Here's how the part is built. I have some questions about the finished solid (model axes, mm). Round coordinates to 2 decimals unless told otherwise and drop trailing zeros. Loops run counter-clockwise (first coordinate to the right, second up) from the corner with the lowest first, then second, coordinate; pieces in that order, holes last. Notation, with made-up numbers: M -31.75,-37.5 L -16.75,-37.5 A29 cw -16.75,-13.5 Z; hole C -12,41 d8. An arc over 180 degrees is marked long. Use a Markdown table: item, result.
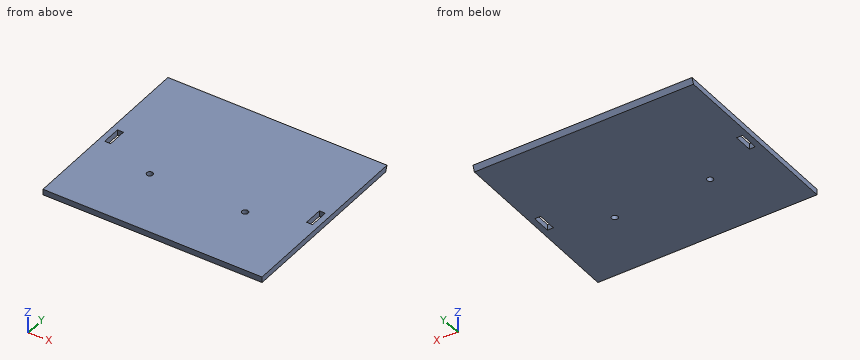
from build123d import *

# Parameters (mm, degrees)
F0_W     = 115
F0_H     = 98
F1_DEPTH = 3
F2_W     = 3.1
F2_H     = 10
F3_DEPTH = 3
F4_SIZE2 = 1.091901
F4_SIZE  = 2.99999
F8_D     = 3.2
F8_DEPTH = 5
F8_TIP   = 0.9613769904


# Not quite as in the source:
# - a fillet or chamfer is up to 0.001 mm smaller than in the source, because OpenCascade refuses the exact size
# - a pattern or mirror of a feature is missing from the dataset's text; its kind, count and spacing are read off the source's solid


with BuildPart() as f1:
    # F0 (on Top) → F1 (new body)
    with BuildSketch(Plane.XY):
        Rectangle(F0_W, F0_H)
    extrude(amount=-F1_DEPTH)

    # F2 (on face) → F3 (cut, through all)
    with BuildSketch(Plane.XY):
        with Locations((53, 0)):
            Rectangle(F2_W, F2_H)
    f3 = extrude(amount=-F3_DEPTH, mode=Mode.SUBTRACT)

    # F3_copies: F3 across plane
    add(f3.mirror(Plane(origin=(0, 0, 0), x_dir=(0, 0, -1), z_dir=(-1, 0, 0))), mode=Mode.SUBTRACT)

    # F4 (size 3 and 1.0919107028 in the source; OpenCascade refuses exactly that, so slightly less here)
    f4_edges = [f1.edges().sort_by_distance(p)[0] for p in [
        (0, 49, -3),
    ]]
    f4_side = f1.faces().sort_by_distance((0, 49, -1.5))[0]
    chamfer(f4_edges, length=F4_SIZE, length2=F4_SIZE2, reference=f4_side)

    # F8
    with Locations(Plane(origin=(0, 0, -3), x_dir=(1, 0, 0), z_dir=(0, 0, -1))):
        with Locations((25, 13.7153716188), (-25, 13.7153716188)):
            Hole(F8_D / 2, depth=F8_DEPTH)
            with Locations((0, 0, -(F8_DEPTH + F8_TIP / 2))):  # 118° drill point
                Cone(0, F8_D / 2, F8_TIP, mode=Mode.SUBTRACT)


solid = f1.part
1. I need wall thicknesses on probe 1 along X at (y, z) = (-15, -2.4); probe 2 along Y at (x, z) = (25, -1.9); probe 3 along Y at (x, z) = (25, -1.1). Which ranges of each line are inside material? Lowest first, please. Write a range as from..to.
Answer sheet:
| item | result |
|---|---|
| probe 1 | -57.5..-25.95, -24.05..24.05, 25.95..57.5 |
| probe 2 | -49..-15.32, -12.12..48.31 |
| probe 3 | -49..-15.32, -12.12..48.6 |
2. Imagine slicing it at B-B, the plane y = 1.5. Write out the boundary of the cut face in (x, z).
Answer sheet:
| item | result |
|---|---|
| outline | M -57.5,-3 L -54.55,-3 L -54.55,0 L -57.5,0 Z; M -51.45,-3 L 51.45,-3 L 51.45,0 L -51.45,0 Z; M 54.55,-3 L 57.5,-3 L 57.5,0 L 54.55,0 Z |
3. For pin 1 Ø0.9 at (x, z) = (-53.5, -2) entering from +Y, with a flat end and sliding along its axis, tell me the tip position at first contact or that it passes through.
Answer sheet:
| item | result |
|---|---|
| pin 1 | y = 48.44 |
